Geometry: see drawing. Coordinates: mm, zero at the bounding-box minimum. A direction names the side the tool comes from. Coordinates: 2 decimals unless noted, no trailing zeros. Order: outer loops, then holes, each group sorted by start corner. A loop starts at its lowest first (then second) coordinate and runs counter-clockwise, first axis right, second up. Notation, with made-up numbers: M -30.75,63 L -0.75,63 A19 ccw -0.75,82 Z; hole C -11,50.25 d8. An arc over 180 degrees is marked long. Answer in a Markdown table with one row per item.
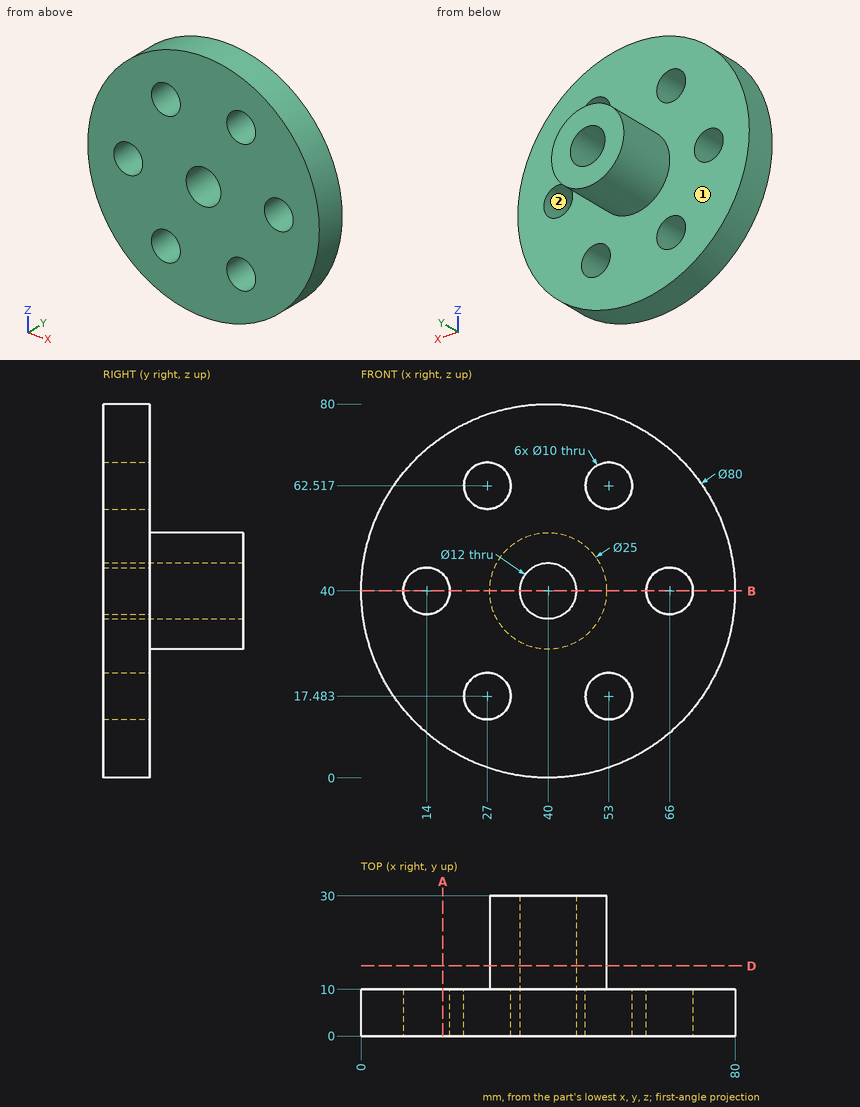
1) Cut plane D-D, the plane y = 15. Output: boundary loops of the cut face in (x, z).
Resolved:
| item | result |
|---|---|
| outline | C 40,40 d25; hole C 40,40 d12 |
2) Contact query for flat-ended pins moving along their axis: pin 1 (6 mm diameter, centred on x = 58, y = 22, fed in from -Z); pin 2 (3 mm diameter, centred on x = 18, z = 37.5, fed in from +Y); pin 3 (1 mm diameter, centred on x = 30.5, y = 23, fed in from -Z) (1 decimal); pin 4 (1.5 mm diameter, centred on x = 29, z = 50, fed in from -Y). Output: stop coordinate, or through.
Resolved:
| item | result |
|---|---|
| pin 1 | passes through |
| pin 2 | stops at y = 10 |
| pin 3 | stops at z = 31.3 |
| pin 4 | stops at y = 0 |
3) Reachability of the marked faces 1 and 2 from +Z, -Z, +X, -X, +Y, -Y: full face, straight path, thin tool, end or side. Return the list, or none.
Resolved:
| item | result |
|---|---|
| face 1 | +Y |
| face 2 | +Y, -Y |
4) Cut plane B-B, the plane z = 40. Output: boundary loops of the cut face in (x, y).
Resolved:
| item | result |
|---|---|
| outline | M 0,0 L 9,0 L 9,10 L 0,10 Z; M 19,0 L 34,0 L 34,30 L 27.5,30 L 27.5,10 L 19,10 Z; M 46,0 L 61,0 L 61,10 L 52.5,10 L 52.5,30 L 46,30 Z; M 71,0 L 80,0 L 80,10 L 71,10 Z |
5) Cut plane A-A, the plane x = 17.5. Output: boundary loops of the cut face in (y, z), and give its area (3 significant figures).
Resolved:
| item | result |
|---|---|
| outline | M 0,6.93 L 10,6.93 L 10,36.43 L 0,36.43 Z; M 0,43.57 L 10,43.57 L 10,73.07 L 0,73.07 Z |
| area | 590 mm2 |
6) Material intervals for probe 1 along X at (y, z) = (1.5, 20.5) (1 decimal); probe 2 along Z at (x, y) = (53, 4.25); probe 3 along Z at (x, y) = (40, 7.25), sorted ascending.
Resolved:
| item | result |
|---|---|
| probe 1 | x = 5.1 to 23, 31 to 49, 57 to 74.9 |
| probe 2 | z = 2.17 to 12.48, 22.48 to 57.52, 67.52 to 77.83 |
| probe 3 | z = 0 to 34, 46 to 80 |
